Could you check a few things on this model? Use its own coordinates, in mm. A direction names the side the tool comes from. Round coordinates to 2 decimals unless told otherwise and drop trailing zeros. Loops run counter-clockwise (first coordinate to the right, second up) from the corner with the lowest first, then second, coordinate; pieces in that order, holes last. Notation, with made-up numbers: (66.5, -31) -> (116.5, -31) arc R25 ccw to (116.5, 6) -> close; hole circle Ø10 at (-35, 45.25). An arc over 180 degrees is marked (long way). Use CSV: the item, a comma, the result in double quotes. Start each with the question number.
```python
from build123d import *

# Parameters (mm, degrees)
F0_W          = 159.512
F0_H          = 80.772
F1_DEPTH      = 9.398
F2_R          = 7.62
F3_R          = 5.08
F5_DEPTH      = 79.757
F5_DEPTH_BACK = 79.757
F6_T          = -2.54
F7_W          = 19.05
F7_H          = 38.1
F8_DEPTH      = 30.48
F9_R          = 5.08


with BuildPart() as f1:
    # F0 (on Top) → F1 (new body)
    with BuildSketch(Plane.XY):
        Rectangle(F0_W, F0_H)
    extrude(amount=F1_DEPTH)

    # F2
    f2_edges = [f1.edges().sort_by_distance(p)[0] for p in [
        (79.756, -40.386, 4.699),
        (79.756, 40.386, 4.699),
        (-79.756, -40.386, 4.699),
        (-79.756, 40.386, 4.699),
    ]]
    fillet(f2_edges, radius=F2_R)

    # F3
    f3_edges = [f1.edges().sort_by_distance(p)[0] for p in [
        (79.756, 0, 9.398),
        (77.524154, -38.154154, 9.398),
        (77.524154, 38.154154, 9.398),
        (0, -40.386, 9.398),
        (0, 40.386, 9.398),
        (-77.524154, -38.154154, 9.398),
        (-77.524154, 38.154154, 9.398),
        (-79.756, 0, 9.398),
    ]]
    fillet(f3_edges, radius=F3_R)

    # F4 (on Right) → F5 (cut, two sides)
    with BuildSketch(Plane.YZ) as f5_sk:
        Polygon((35.306, 0), (40.386, 0), (40.386, 2.54), align=None)
        Polygon((-40.386, 0), (-35.306, 0), (-40.386, 2.54), align=None)
    extrude(amount=F5_DEPTH, mode=Mode.SUBTRACT)
    extrude(f5_sk.sketch, amount=-F5_DEPTH_BACK, mode=Mode.SUBTRACT)

    # F6
    f6_openings = [f1.faces().sort_by_distance(p)[0] for p in [
        (0, -37.816494, 1.255247),
        (0, 37.816494, 1.255247),
        (0, 0, 0),
    ]]
    offset(amount=F6_T, openings=f6_openings)

    # F7 (on Top) → F8 (cut)
    with BuildSketch(Plane.XY):
        with Locations((-52.451, 3.556)):
            Rectangle(F7_W, F7_H)
    extrude(amount=F8_DEPTH, mode=Mode.SUBTRACT)

    # F9
    f9_edges = [f1.edges().sort_by_distance(p)[0] for p in [
        (-61.976, -15.494, 8.128),
        (-42.926, -15.494, 8.128),
        (-61.976, 22.606, 8.128),
        (-42.926, 22.606, 8.128),
    ]]
    fillet(f9_edges, radius=F9_R)


solid = f1.part
```
1. Suppose I cut it at C-C (x = 50.5). List the corners of the cut face in (y, z) for me, then the cut area to 3 significant figures.
2. We'd pull the mould along X, two halves only. Please class faces 1 (the face through (78.33, -37.205, 2.669)), 2 (the face through (-75.767, 36.318, 2.189)), 3 (the face through (-79.756, 0, 2)), 4 (the face through (77.216, 0, 2)): pulls with the +X half, pulls with the -X half, needs draft (parallel to the pull), parting line crosses it, or undercut.
3. For faces 5 (the face through (-77.216, 0, 2)), 6 (the face through (-60.527, -13.966, 8.146)), 7 (the face through (1.11, -38.939, 1.817)), which set-ups out of +Z, -Z, +X, -X, +Y, -Y let a thin tool reach every point of the face, with its end or its side?
4. Suppose I cut it at A-A (y = -5). List the corners of the cut face in (x, z) for me.
5. Suppose I cut it at B-B (y = -22.5). List the corners of the cut face in (x, z) for me.
6. Will these pins go through, and if not, where does the flat tip stop? pin 1 (8 mm diameter, centred on x = -53.5, y = 15.5, fed in from -Z); pin 2 (5 mm diameter, centred on y = 31, z = 8, fed in from +X); pin 3 (0.8 mm diameter, centred on y = 2.5, z = 7.5, fed in from +X); pin 4 (1.3 mm diameter, centred on x = -51, z = 8, fed in from -Y).
7. If I drill on L1, parallel to X at y = 25, z = 3.5; L2, parallel to Z at x = 16, y = 25; L3, parallel to Y at x = -68, z = 3.5, over which ranges is the centre line in solid material (lowest first)?
Geometry check:
1,outline,"(-40.39, 2.54) -> (-37.85, 1.27) -> (-37.85, 4.32) arc R2.54 cw to (-35.31, 6.86) -> (35.31, 6.86) arc R2.54 cw to (37.85, 4.32) -> (37.85, 1.27) -> (40.39, 2.54) -> (40.39, 4.32) arc R5.08 ccw to (35.31, 9.4) -> (-35.31, 9.4) arc R5.08 ccw to (-40.39, 4.32) -> close"
1,area,"222 mm²"
2,face 1,"pulls with the +X half"
2,face 2,"undercut"
2,face 3,"pulls with the -X half"
2,face 4,"undercut"
3,face 5,"-Z"
3,face 6,"+Z, -Z"
3,face 7,"-Z, +X, -X, -Y"
4,outline,"(-79.76, 0) -> (-77.22, 0) -> (-77.22, 4.32) arc R2.54 cw to (-74.68, 6.86) -> (-61.98, 6.86) -> (-61.98, 9.4) -> (-74.68, 9.4) arc R5.08 ccw to (-79.76, 4.32) -> close; (-42.93, 6.86) -> (74.68, 6.86) arc R2.54 cw to (77.22, 4.32) -> (77.22, 0) -> (79.76, 0) -> (79.76, 4.32) arc R5.08 ccw to (74.68, 9.4) -> (-42.93, 9.4) -> close"
5,outline,"(-79.76, 0) -> (-77.22, 0) -> (-77.22, 4.32) arc R2.54 cw to (-74.68, 6.86) -> (74.68, 6.86) arc R2.54 cw to (77.22, 4.32) -> (77.22, 0) -> (79.76, 0) -> (79.76, 4.32) arc R5.08 ccw to (74.68, 9.4) -> (-74.68, 9.4) arc R5.08 ccw to (-79.76, 4.32) -> close"
6,pin 1,"passes through"
6,pin 2,"stops at x = 79.62"
6,pin 3,"stops at x = 78.93"
6,pin 4,"stops at y = -39.38"
7,L1,"x = -79.76 to -77.22, 77.22 to 79.76"
7,L2,"z = 6.86 to 9.4"
7,L3,"y = -40.39 to -37.85, 37.85 to 40.39"
